Build history of the part. All positions in model axes, mm. A direction names the side the tool comes from. Round coordinates to 2 decimals unless told otherwise and drop trailing zeros. Write each loop counter-clockwise with the first axis right and the second up, starting at its lowest first coordinate (ties: lowest second). Pieces come first, ordered by that corner, then holes. Notation, with made-up numbers: M -5.5,41 L 18.5,41 A15 cw 18.5,53 Z; hole C -36,-31.75 d8. An arc over 180 degrees is marked long. One line per item, written item: value. Start each with the question number.
Autodesk Inventor part; units mm, degrees
ref_plane "YZ Plane" through (0, 0, 0) normal (1, 0, 0) x (0, 1, 0)
ref_plane "XZ Plane" through (0, 0, 0) normal (0, 1, 0) x (-1, 0, 0)
ref_plane "XY Plane" through (0, 0, 0) normal (0, 0, 1) x (1, 0, 0)
sketch "Sketch1" plane through (0, 0, 0) normal (0, 0, 1) x (1, 0, 0)
  circle A0 centre (0, 0) radius 2.5
  dimension "d0" = 5
extrude "Extrusion1" add sketch "Sketch1" along normal blind 10
sketch "Sketch2" plane through (0, 0, 10) normal (0, 0, 1) x (1, 0, 0)
  circle A0 centre (0, 0) radius 2.5
  circle A1 centre (0, 0) radius 1
  dimension "d3" = 2
extrude "Extrusion2" add sketch "Sketch2" along normal blind 3 contours A1
sketch "Sketch3" plane through (0, 0, 0) normal (0, 0, -1) x (-1, 0, 0)
  circle A0 centre (0, 0) radius 1
  dimension "d6" = 2
extrude "Extrusion3" add sketch "Sketch3" along normal blind 3
properties part number "Bone-1cm"
Item 1: Cut at D-D, the plane z = -1. Write the cut outline in (x, y), plus the area to 3 significant figures.
Item 2: Cut at C-C, the plane z = 4.25. Write the cut outline in (x, y), plus the area to 3 significant figures.
Item 3: Which spindle directions (+Z, -Z, +X, -X, +Y, -Y) get a long thin tool onto all of the face, cutting with end or side? Do faces 1 (the flat face through (1, -1, 0)), 2 (the cylindrical face through (0, 1, 11)), 3 (the flat face through (0, 0, 13)). Say none if no direction does.
Item 4: Drill centre lines: line 1 (Z direction, x = 0.7, y = -1.95); line 2 (Y direction, x = -0.1, z = 8.75); line 3 (X direction, y = 0.05, z = -1). Where is each one in solid material? Low to high.
Item 5: Cut at A-A, the plane y = 0. Write the cut outline in (x, z).
Computed values:
1. outline: C 0,0 d2
1. area: 3.14 mm2
2. outline: C 0,0 d5
2. area: 19.6 mm2
3. face 1: -Z
3. face 2: +Z
3. face 3: +Z, +X, -X, +Y, -Y
4. line 1: z = 0 to 10
4. line 2: y = -2.5 to 2.5
4. line 3: x = -1 to 1
5. outline: M -2.5,0 L -1,0 L -1,-3 L 1,-3 L 1,0 L 2.5,0 L 2.5,10 L 1,10 L 1,13 L -1,13 L -1,10 L -2.5,10 Z
